Verification items for the finished model (mm, model axes). Face numbers are marked on the shaded views. A direction names the side the tool comes from. Coordinates: 2 decimals unless noted, no trailing zeros. Loops run counter-clockwise (first coordinate to the right, second up) from the corner with the lowest first, then second, coordinate; pieces in that order, holes last. Notation, with made-up numbers: (-3.5, 81) -> (5.5, 81) arc R27 ccw to (5.5, 97) -> close; hole circle Ø3 at (-4, 19). An arc over 180 degrees is marked (long way). Answer as a JSON object with one key per item and string values. Group by question number.
Q1. Gauge pin test, flat ends, axial feed: pin 1 Ø4 at (x, y) = (-41.5, -3) entering from -Z; pin 2 Ø10 at (y, z) = (-7.5, 53) entering from +X; pin 3 Ø5 at (y, z) = (-15.5, 26.5) entering from +X. Record the tip position at first contact, or that the pin passes through.
Q2. Cross-section at C-C on y = -6.25. Record the boundary of the cut face in (x, z).
Q3. Scan lines: L1, parallel to Z at x = -42.5, y = -17.75; L2, parallel to Z at x = -37.5, y = -10.25; L3, parallel to X at y = -3.5, z = 36. Record each from-to range of solid material in increasing order.
Q4. Set-up check for the marked faces 1 and 2: record each of +Z, -Z, +X, -X, +Y, -Y from which the full face is reachable in a straight line by a thin tool's end or side.
Q5. Cross-section at A-A on x = -36. Record the boundary of the cut face in (y, z).
Q6. Release check for a two-part mould opening along Z. For the marked faces 3, 4, 5 and 6 record: released by +Z, released by -Z, zero draft, split by the parting line, or undercut.
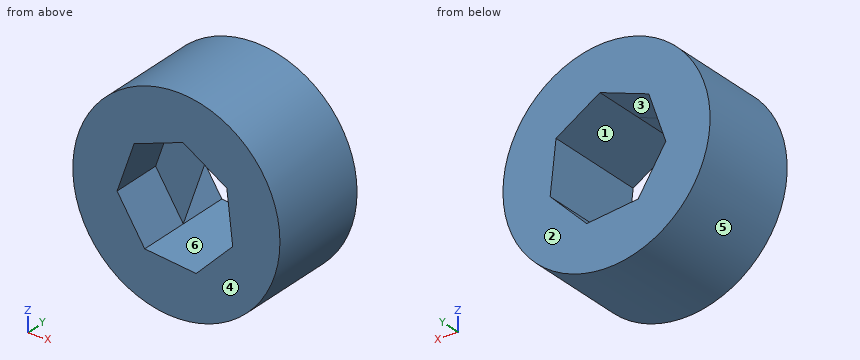
```python
from build123d import *

# Parameters (mm, degrees)
F0_R     = 25.4
F1_DEPTH = 25.4
F3_DEPTH = 12.7
F4_DEPTH = 50.8


with BuildPart() as f1:
    # F0 (on Front) → F1 (new body)
    with BuildSketch(Plane.XZ):
        with Locations((-42.658649, 34.146946)):
            Circle(F0_R)
    extrude(amount=F1_DEPTH)

    # F2 (on face) → F3 (cut)
    with BuildSketch(Plane.XZ.offset(25.4)):
        Polygon((-53.026801, 44.476137), (-57.198773, 32.480944), (-50.421735, 21.740285), (-37.798936, 20.342094), (-28.8356, 29.339239), (-30.281302, 41.956685), (-41.047399, 48.693238), align=None)
    extrude(amount=-F3_DEPTH, mode=Mode.SUBTRACT)

    # F3_face (on face) → F4 (cut)
    with BuildSketch(Plane(origin=(-42.658649, -12.7, 34.146946), x_dir=(1, 0, 0), z_dir=(0, -1, 0))):
        Polygon((12.377347, 7.809739), (1.61125, 14.546292), (-10.368151, 10.329191), (-14.540123, -1.666002), (-7.763086, -12.406661), (4.859713, -13.804852), (13.823049, -4.807707), align=None)
    extrude(amount=-F4_DEPTH, mode=Mode.SUBTRACT)


solid = f1.part
```
Computed values:
{
 "1": {"pin 1": "stops at z = 8.75", "pin 2": "stops at x = -21.37", "pin 3": "stops at x = -17.79"},
 "2": {"outline": "circle Ø50.8 at (-42.66, 34.15); hole (-57.2, 32.48) -> (-50.42, 21.74) -> (-37.8, 20.34) -> (-28.84, 29.34) -> (-30.28, 41.96) -> (-41.05, 48.69) -> (-53.03, 44.48) -> close"},
 "3": {"L1": "z = 8.75 to 20.86, 48.18 to 59.55", "L2": "z = 9.28 to 20.64, 46.47 to 59.02", "L3": "x = -67.99 to -55.97, -29.6 to -17.33"},
 "4": {"face 1": "+Y, -Y", "face 2": "+Z, -Z, +X, -X, +Y"},
 "5": {"outline": "(-25.4, 9.64) -> (0, 9.64) -> (0, 22.15) -> (-25.4, 22.15) -> close; (-25.4, 45.53) -> (0, 45.53) -> (0, 58.66) -> (-25.4, 58.66) -> close"},
 "6": {"face 3": "undercut", "face 4": "zero draft", "face 5": "split by the parting line", "face 6": "undercut"}
}
